```python
from build123d import *

# Parameters (mm, degrees)
BOX005_W          = 70
BOX005_H          = 10
BOX005_DEPTH      = 30
BOX006_W          = 35
BOX006_H          = 10
BOX006_DEPTH      = 25
BOX007_W          = 35
BOX007_H          = 10
BOX007_DEPTH      = 36
BOX008_W          = 85
BOX008_H          = 10
BOX008_DEPTH      = 50
BOX009_W          = 22
BOX009_H          = 10
BOX009_DEPTH      = 35
BOX004_W          = 110
BOX004_H          = 10
BOX004_DEPTH      = 36
CYLINDER008_R     = 2
CYLINDER008_DEPTH = 10
CYLINDER009_R     = 2
CYLINDER009_DEPTH = 10
CYLINDER010_R     = 2
CYLINDER010_DEPTH = 10
CYLINDER011_R     = 2
CYLINDER011_DEPTH = 10
CYLINDER005_R     = 1.6
CYLINDER005_DEPTH = 10
CYLINDER007_R     = 1.6
CYLINDER007_DEPTH = 10
CYLINDER004_R     = 1.6
CYLINDER004_DEPTH = 10
CYLINDER006_R     = 1.6
CYLINDER006_DEPTH = 10
BOX_W             = 160
BOX_H             = 1.6
BOX_DEPTH         = 100
BOX001_W          = 155
BOX001_H          = 2.9
BOX001_DEPTH      = 100


with BuildPart() as cuts002:
    # Box005 → Box005 (new body)
    with BuildSketch(Plane(origin=(90, 10, 14.6), x_dir=(1, 0, 0), z_dir=(0, 0, 1))):
        with Locations((35, 5)):
            Rectangle(BOX005_W, BOX005_H)
    extrude(amount=BOX005_DEPTH)


with BuildPart() as cuts003:
    # Box006 → Box006 (new body)
    with BuildSketch(Plane(origin=(0, 10, 14.6), x_dir=(1, 0, 0), z_dir=(0, 0, 1))):
        with Locations((17.5, 5)):
            Rectangle(BOX006_W, BOX006_H)
    extrude(amount=BOX006_DEPTH)


with BuildPart() as cuts004:
    # Box007 → Box007 (new body)
    with BuildSketch(Plane(origin=(0, 10, 54.2), x_dir=(1, 0, 0), z_dir=(0, 0, 1))):
        with Locations((17.5, 5)):
            Rectangle(BOX007_W, BOX007_H)
    extrude(amount=BOX007_DEPTH)


with BuildPart() as cuts005:
    # Box008 → Box008 (new body)
    with BuildSketch(Plane(origin=(75, 10, 54), x_dir=(1, 0, 0), z_dir=(0, 0, 1))):
        with Locations((42.5, 5)):
            Rectangle(BOX008_W, BOX008_H)
    extrude(amount=BOX008_DEPTH)


with BuildPart() as cuts006:
    # Box009 → Box009 (new body)
    with BuildSketch(Plane(origin=(50, 10, 4), x_dir=(1, 0, 0), z_dir=(0, 0, 1))):
        with Locations((11, 5)):
            Rectangle(BOX009_W, BOX009_H)
    extrude(amount=BOX009_DEPTH)


with BuildPart() as cuts:
    # Box004 → Box004 (new body)
    with BuildSketch(Plane(origin=(50, 10, 54), x_dir=(1, 0, 0), z_dir=(0, 0, 1))):
        with Locations((55, 5)):
            Rectangle(BOX004_W, BOX004_H)
    extrude(amount=BOX004_DEPTH)

    # Fusion005: union cuts002, cuts003, cuts004, cuts005, cuts006
    add(cuts002.part)
    add(cuts003.part)
    add(cuts004.part)
    add(cuts005.part)
    add(cuts006.part)


with BuildPart() as m2s008:
    # Cylinder008 → Cylinder008 (new body)
    with BuildSketch(Plane(origin=(9, 0, 47.5), x_dir=(1, 0, 0), z_dir=(0, -1, 0))):
        Circle(CYLINDER008_R)
    extrude(amount=CYLINDER008_DEPTH)


with BuildPart() as m2s009:
    # Cylinder009 → Cylinder009 (new body)
    with BuildSketch(Plane(origin=(67, 0, 47.5), x_dir=(1, 0, 0), z_dir=(0, -1, 0))):
        Circle(CYLINDER009_R)
    extrude(amount=CYLINDER009_DEPTH)


with BuildPart() as m2s010:
    # Cylinder010 → Cylinder010 (new body)
    with BuildSketch(Plane(origin=(67, 0, 96.5), x_dir=(1, 0, 0), z_dir=(0, -1, 0))):
        Circle(CYLINDER010_R)
    extrude(amount=CYLINDER010_DEPTH)


with BuildPart() as c1cuts:
    # Cylinder011 → Cylinder011 (new body)
    with BuildSketch(Plane(origin=(9, 0, 96.5), x_dir=(1, 0, 0), z_dir=(0, -1, 0))):
        Circle(CYLINDER011_R)
    extrude(amount=CYLINDER011_DEPTH)

    # Fusion003: union m2s008, m2s009, m2s010
    add(m2s008.part)
    add(m2s009.part)
    add(m2s010.part)


with BuildPart() as c1cuts_1:
    # Fusion003 placement: moved
    add(c1cuts.part.moved(Location((0, 16.4, 0))))


with BuildPart() as m2s005:
    # Cylinder005 → Cylinder005 (new body)
    with BuildSketch(Plane(origin=(14, 0, 20), x_dir=(1, 0, 0), z_dir=(0, -1, 0))):
        Circle(CYLINDER005_R)
    extrude(amount=CYLINDER005_DEPTH)


with BuildPart() as m2s007:
    # Cylinder007 → Cylinder007 (new body)
    with BuildSketch(Plane(origin=(49, 0, 20), x_dir=(1, 0, 0), z_dir=(0, -1, 0))):
        Circle(CYLINDER007_R)
    extrude(amount=CYLINDER007_DEPTH)


with BuildPart() as m2s004:
    # Cylinder004 → Cylinder004 (new body)
    with BuildSketch(Plane(origin=(49, 0, 3), x_dir=(1, 0, 0), z_dir=(0, -1, 0))):
        Circle(CYLINDER004_R)
    extrude(amount=CYLINDER004_DEPTH)


with BuildPart() as basecuts:
    # Cylinder006 → Cylinder006 (new body)
    with BuildSketch(Plane(origin=(14, 0, 3), x_dir=(1, 0, 0), z_dir=(0, -1, 0))):
        Circle(CYLINDER006_R)
    extrude(amount=CYLINDER006_DEPTH)

    # Fusion002: union m2s005, m2s007, m2s004
    add(m2s005.part)
    add(m2s007.part)
    add(m2s004.part)


with BuildPart() as basecuts_1:
    # Fusion002 placement: moved
    add(basecuts.part.moved(Location((30, 16.2, 15))))

    # Fusion004: union c1Cuts
    add(c1cuts_1.part)


with BuildPart() as base:
    # Box → Box (new body)
    with BuildSketch(Plane(origin=(0, 14.6, 4), x_dir=(1, 0, 0), z_dir=(0, 0, 1))):
        with Locations((80, 0.8)):
            Rectangle(BOX_W, BOX_H)
    extrude(amount=BOX_DEPTH)


with BuildPart() as cut002:
    # Box001 → Box001 (new body)
    with BuildSketch(Plane(origin=(2.5, 11.7, 4), x_dir=(1, 0, 0), z_dir=(0, 0, 1))):
        with Locations((77.5, 1.45)):
            Rectangle(BOX001_W, BOX001_H)
    extrude(amount=BOX001_DEPTH)

    # Fusion001: union base
    add(base.part)

    # Cut001: cut baseCuts
    add(basecuts_1.part, mode=Mode.SUBTRACT)

    # Cut002: cut cuts
    add(cuts.part, mode=Mode.SUBTRACT)


solid = cut002.part
```
Here's how the part is built. I have some questions about the finished solid (model axes, mm). A direction names the side the tool comes from. Give positions to 0.01 mm unless a question says otherwise; leave off trailing zeros. Write each loop counter-clockwise with the first axis right and the second up, starting at its lowest first coordinate (ties: lowest second). Pieces come first, ordered by that corner, then holes.
(1) On a 3-axis mill with a long thin cutter (end or side, diameter ignored), from which of +Z, -Z, +X, -X, +Y, -Y can I reach the whole of each face in a straight line? I mean faces 4 (the face through (61, 14, 39)), 5 (the face through (17, 14, 39.6)), 6 (the face through (2.5, 13, 47)). Say none if no direction works.
Output values:
face 4: -Z, +Y, -Y
face 5: -X, +Y, -Y
face 6: +Z, -Z, -X, -Y
(2) Imagine slicing it at D-D, the plane z = 18. Write out the boundary of the cut face in (x, y).
Output values:
outline: (35, 11.7) - (42.4, 11.7) - (42.4, 16.2) - (35, 16.2) - close; (45.6, 11.7) - (50, 11.7) - (50, 16.2) - (45.6, 16.2) - close; (72, 11.7) - (77.4, 11.7) - (77.4, 16.2) - (72, 16.2) - close; (80.6, 11.7) - (90, 11.7) - (90, 16.2) - (80.6, 16.2) - close
(3) Imagine slicing it at A-A, the plane z = 47.5. Write out the boundary of the cut face in (x, y), and give its area (4 significant figures).
Output values:
outline: (0, 14.6) - (2.5, 14.6) - (2.5, 11.7) - (7, 11.7) - (7, 16.2) - (0, 16.2) - close; (11, 11.7) - (65, 11.7) - (65, 16.2) - (11, 16.2) - close; (69, 11.7) - (157.5, 11.7) - (157.5, 14.6) - (160, 14.6) - (160, 16.2) - (69, 16.2) - close
area: 669.5 mm2
(4) Imagine slicing it at B-B, the plane x = 67. Write out the boundary of the cut face in (y, z), and give its area (3 significant figures).
Output values:
outline: (11.7, 39) - (16.2, 39) - (16.2, 45.5) - (11.7, 45.5) - close; (11.7, 49.5) - (16.2, 49.5) - (16.2, 54) - (11.7, 54) - close; (11.7, 90) - (16.2, 90) - (16.2, 94.5) - (11.7, 94.5) - close; (11.7, 98.5) - (16.2, 98.5) - (16.2, 104) - (11.7, 104) - close
area: 94.5 mm2
(5) If I drill on L1, parallel to Z at x = 9, y = 13.5; L2, parallel to Z at x = 79, y = 15.1; L3, parallel to Z at x = 114, y = 13.1, over which ranges is the centre line in solid material (lowest first)?
Output values:
L1: z = 4 to 14.6, 39.6 to 45.5, 49.5 to 54.2, 90.2 to 94.5, 98.5 to 104
L2: z = 4 to 16.4, 19.6 to 33.4, 36.6 to 54
L3: z = 4 to 14.6, 44.6 to 54
(6) Thinking about a two-plate mould opening in Z: for faces 1 (the face through (43.792, 13.981, 19.586)), 2 (the face through (37, 14, 104)), 3 (the face through (157.5, 13, 49)), which applies, pulls with the +Z half, pulls with the -Z half, needs draft (parallel to the pull), parting line crosses it, or undercut?
Output values:
face 1: undercut
face 2: pulls with the +Z half
face 3: needs draft
(7) Imagine slicing it at C-C, the plane y = 12.5. Count the separate pieces of the cut face and the enclosed holes in it, and give its area (3 significant figures).
Output values:
separate pieces: 1
enclosed holes: 8
area: 5,620 mm2
(8) Will these pins go through, and if not, where does the flat tip stop? pin 1 (1.4 mm diameter, centred on y = 12.5, z = 47, fed in from -X); pin 2 (2 mm diameter, centred on x = 159, z = 51.5, fed in from -Y); pin 3 (1.4 mm diameter, centred on y = 13.5, z = 8.5, fed in from +X).
Output values:
pin 1: stops at x = 2.5
pin 2: stops at y = 14.6
pin 3: stops at x = 157.5
